Work out the finished part from the listing and answer in its coordinate system (mm). A direction names the side the tool comes from. Round coordinates to 2 decimals unless told otherwise and drop trailing zeros. Write each loop counter-clockwise with the first axis right and the second up, starting at its lowest first coordinate (ties: lowest second). Pieces come first, ordered by that corner, then holes. Notation, with made-up numbers: (43.5, 65) -> (59.5, 65) arc R24 ccw to (59.5, 79) -> close; hole circle Ø1 at (-6.75, -3). An arc over 180 degrees is marked (long way). One line per item, written item: value.
```python
from build123d import *

# Parameters (mm, degrees)
SALIENTE_EXTRUIR1_DEPTH = 15
CROQUIS3_W              = 27
CROQUIS3_H              = 10
CORTAR_EXTRUIR1_DEPTH   = 103
CROQUIS2_R              = 1.75
CORTAR_EXTRUIR2_DEPTH   = 25.85
CROQUIS4_R              = 2.5
CROQUIS4_R_2            = 2.643656248
CORTAR_EXTRUIR3_DEPTH   = 34


with BuildPart() as part:
    # Croquis1 → Saliente-Extruir1 (new body)
    with BuildSketch(Plane(origin=(0, 0, 0), x_dir=(1, 0, 0), z_dir=(0, 1, 0))):
        with BuildLine():
            Line((10.672482707, -9.762077578), (7.472477359, -9.762077578))
            ThreePointArc((7.472477359, -9.762077578), (5.351157015, -8.883397922), (4.472477359, -6.762077578))
            Line((4.472477359, -6.762077578), (4.472477359, 6.050505251))
            ThreePointArc((4.472477359, 6.050505251), (5.354589632, 8.175252666), (7.48217841, 9.050489566))
            Line((7.48217841, 9.050489566), (10.672482707, 9.040173078))
            Line((10.672482707, 9.040173078), (10.672482707, 32.133052813))
            Line((10.672482707, 32.133052813), (-23.183050508, 32.133052813))
            Line((-23.183050508, 32.133052813), (-23.183050508, -32.8682401))
            Line((-23.183050508, -32.8682401), (10.672482707, -32.8682401))
            Line((10.672482707, -32.8682401), (10.672482707, -9.762077578))
        make_face()
    extrude(amount=SALIENTE_EXTRUIR1_DEPTH)

    # Croquis3 → Cortar-Extruir1 (cut)
    with BuildSketch(Plane(origin=(0, 0, -32.133052813), x_dir=(-1, 0, 0), z_dir=(0, 0, -1))):
        with Locations((9.683050508, 10)):
            Rectangle(CROQUIS3_W, CROQUIS3_H)
    extrude(amount=-CORTAR_EXTRUIR1_DEPTH, mode=Mode.SUBTRACT)

    # Croquis2 → Cortar-Extruir2 (cut)
    with BuildSketch(Plane.XZ):
        with Locations(Location((0.416949492, -7.282406356, 0), (0, 0, 270))):
            Circle(CROQUIS2_R)
        with Locations(Location((-19.583050508, -7.282406356, 0), (0, 0, 270))):
            Circle(CROQUIS2_R)
        with Locations((-19.583050508, 8.017593644)):
            Circle(CROQUIS2_R)
        with Locations((0.416949492, 8.017593644)):
            Circle(CROQUIS2_R)
    extrude(amount=-CORTAR_EXTRUIR2_DEPTH, mode=Mode.SUBTRACT)

    # Croquis4 → Cortar-Extruir3 (cut)
    with BuildSketch(Plane(origin=(10.672482707, 0, 0), x_dir=(0, 0, -1), z_dir=(1, 0, 0))):
        with Locations((24.573974701, 7.201679741)):
            Circle(CROQUIS4_R)
        with Locations((-25.426025299, 7.201679741)):
            Circle(CROQUIS4_R_2)
    extrude(amount=-CORTAR_EXTRUIR3_DEPTH, mode=Mode.SUBTRACT)


solid = part.part
```
(1) A tool of negligible diameter and unlimited length cuts with its end or side. For faces 4 (the face through (10.672, 7, -20)), 5 (the face through (-9, 5, -29)), 6 (the face through (4.472, 7, 0)), from which of +Z, -Z, +X, -X, +Y, -Y can it reach the whole face along a straight path? Write none if from no direction.
Reported:
face 4: +Z, -Z, +X, +Y, -Y
face 5: +Z, -Z, -X, +Y
face 6: +X, +Y, -Y
(2) Find section B-B on y = 12. Give the vertices of the cut face in (x, z).
Reported:
outline: (3.82, -32.13) -> (10.67, -32.13) -> (10.67, -9.04) -> (7.48, -9.05) arc R3 cw to (4.47, -6.05) -> (4.47, 6.76) arc R3 cw to (7.47, 9.76) -> (10.67, 9.76) -> (10.67, 32.87) -> (3.82, 32.87) -> close
(3) For a pull along X with two mould halves and no side action, classify faces 1 (the face through (5.375, 7.395, 8.907)), 2 (the face through (0.494, 2.465, -5.534)), 3 (the face through (1.51, 4.76, -24.03)) as pulls with the +X half, pulls with the -X half, needs draft (parallel to the pull), parting line crosses it, or undercut.
Reported:
face 1: pulls with the +X half
face 2: undercut
face 3: needs draft
(4) Find section A-A on y = 8.25. Give the vertices of the cut face in (x, z), plus the area to 3 significant figures.
Reported:
outline: (3.82, -32.13) -> (10.67, -32.13) -> (10.67, -26.84) -> (3.82, -26.84) -> close; (3.82, -22.3) -> (10.67, -22.3) -> (10.67, -9.04) -> (7.48, -9.05) arc R3 cw to (4.47, -6.05) -> (4.47, 6.76) arc R3 cw to (7.47, 9.76) -> (10.67, 9.76) -> (10.67, 23) -> (3.82, 23) -> close; (3.82, 27.85) -> (10.67, 27.85) -> (10.67, 32.87) -> (3.82, 32.87) -> close
area: 268 mm2
(5) Consider probe 1 along Z at (x, y) = (9, 11.25); probe 2 along Z at (x, y) = (5, 5.25); probe 3 along Z at (x, y) = (-18, 3.5). Determine where each line is inside the solid, lowest interval first.
Reported:
probe 1: z = -32.13 to -9.05, 9.76 to 32.87
probe 2: z = -32.13 to -26.14, -23.01 to -7.75, 8.46 to 23.64, 27.21 to 32.87
probe 3: z = -32.13 to -8.03, -6.54 to 7.27, 8.76 to 32.87
(6) Find section C-C on x = -10. Give the vertices of the cut face in (y, z).
Reported:
outline: (0, -32.13) -> (5, -32.13) -> (5, -25.76) arc R2.5 cw to (5, -23.39) -> (5, 23.96) arc R2.64 cw to (5, 26.89) -> (5, 32.87) -> (0, 32.87) -> close
(7) Flat-ended cylindrical pins translate along their axes: pin 1 Ø5 at (y, z) = (8.5, -9) entering from -X; pin 2 Ø5 at (x, z) = (-5, -29.5) entering from +Y. Find the tip coordinate at first contact, or state that the pin passes through.
Reported:
pin 1: stops at x = 3.82
pin 2: stops at y = 5
(8) Find section D-D on z = 14.5. Give the vertices of the cut face in (x, y), plus the area to 3 significant figures.
Reported:
outline: (-23.18, 0) -> (10.67, 0) -> (10.67, 15) -> (3.82, 15) -> (3.82, 5) -> (-23.18, 5) -> close
area: 238 mm2
